Design review of the part built by this model. Coordinates are the model's own, in mm. A direction names the side the tool comes from. Coordinates: 2 decimals unless noted, no trailing zeros. Loops run counter-clockwise (first coordinate to the right, second up) from the corner with the lowest first, then second, coordinate; pieces in that order, holes last. Notation, with made-up numbers: M -8.5,-33.5 L 13.5,-33.5 A7 ccw 13.5,-25.5 Z; hole C 80,5.5 d6. An arc over 180 degrees is marked long. One line per item, written item: value.
```python
from build123d import *

# Parameters (mm, degrees)
F0_R     = 10.16
F1_DEPTH = 50.8
F3_R     = 3.175
F2_W     = 38.1
F2_H     = 15.875
F5_DEPTH = 31.751
F5_TAPER = 12
F6_DEPTH = 25.4


with BuildPart() as f1:
    # F0 (on Top) → F1 (new body)
    with BuildSketch(Plane.XY):
        with BuildLine():
            ThreePointArc((0, 15.875), (11.2253201513, 11.2253201513), (15.875, 0))
            ThreePointArc((15.875, 0), (15.8438414877, -0.9941387788), (15.7504882631, -1.9843750839))
            ThreePointArc((15.7504882631, -1.9843750839), (18.9005858967, 3.968749972), (25.2007812379, 6.35))
            Line((25.2007812379, 6.35), (47.625, 6.35))
            ThreePointArc((47.625, 6.35), (52.1151280605, 4.4901280605), (53.975, 0))
            Line((53.975, 0), (53.975, -12.7))
            ThreePointArc((53.975, -12.7), (54.9049359697, -14.9450640303), (57.15, -15.875))
            Line((57.15, -15.875), (60.325, -15.875))
            ThreePointArc((60.325, -15.875), (62.5700640303, -14.9450640303), (63.5, -12.7))
            Line((63.5, -12.7), (63.5, 3.175))
            ThreePointArc((63.5, 3.175), (59.7802561211, 12.1552561211), (50.8, 15.875))
            Line((50.8, 15.875), (0, 15.875))
        make_face()
        with BuildLine():
            ThreePointArc((15.7504882631, -1.9843750839), (15.8438414877, -0.9941387788), (15.875, 0))
            ThreePointArc((15.875, 0), (11.2253201513, 11.2253201513), (0, 15.875))
            ThreePointArc((0, 15.875), (-11.906250028, -10.5003254841), (15.7504882631, -1.9843750839))
        make_face()
        with Locations((0, 1.905)):
            Circle(F0_R, mode=Mode.SUBTRACT)
    extrude(amount=F1_DEPTH)

    # F3
    f3_edges = [f1.edges().sort_by_distance(p)[0] for p in [
        (25.4, 15.875, 0),
        (25.4, 15.875, 50.8),
    ]]
    fillet(f3_edges, radius=F3_R)

    # F2 (on face) → F5 (cut, through all)
    with BuildSketch(Plane(origin=(0, 15.875, 0), x_dir=(-1, 0, 0), z_dir=(0, 1, 0))):
        with BuildLine():
            ThreePointArc((-7.9375, 33.3375), (-15.875, 25.4), (-7.9375, 17.4625))
            Line((-7.9375, 17.4625), (0, 17.4625))
            Line((0, 17.4625), (0, 33.3375))
            Line((0, 33.3375), (-7.9375, 33.3375))
        make_face()
        with Locations((19.05, 25.4)):
            Rectangle(F2_W, F2_H)
    extrude(amount=-F5_DEPTH, taper=F5_TAPER, mode=Mode.SUBTRACT)

    # F4 (on face) → F6 (cut)
    with BuildSketch(Plane.XZ.offset(15.875)):
        with BuildLine():
            Line((-38.1, 21.828125), (7.9375, 21.828125))
            ThreePointArc((7.9375, 21.828125), (11.509375, 25.4), (7.9375, 28.971875))
            Line((7.9375, 28.971875), (-38.1, 28.971875))
            Line((-38.1, 28.971875), (-38.1, 21.828125))
        make_face()
    extrude(amount=-F6_DEPTH, mode=Mode.SUBTRACT)


solid = f1.part
```
(1) We need section A-A on x = 33. State the section outline as (y, z) points (3 decimals).
Reply:
outline: M 6.35,3.175 A3.175 ccw 9.525,0 L 12.7,0 A3.175 ccw 15.875,3.175 L 15.875,47.625 A3.175 ccw 12.7,50.8 L 9.525,50.8 A3.175 ccw 6.35,47.625 Z
(2) To check wall thickness, follow line 1 along Y through (x, z) = (0, 43) (3 decimals); line 2 along X through (y, z) = (-1, 48.5); line 3 along X through (y, z) = (-2, 6.5) (3 decimals). State the ranges of each line that lie inside material, in increasing order. Write a range as [from, to].
Reply:
line 1: y = [-15.875, -8.255], [12.065, 15.875]
line 2: x = [-15.72, -9.74], [9.74, 15.8], [54.1, 63.38]
line 3: x = [-15.749, -9.38], [9.38, 15.749], [53.975, 63.5]
(3) Tool access review of faces 1 (the cylindrical face through (4.688, -7.109, 10.761)), 2 (the cylindrical face through (54.88, -6.439, 49.845)), 3 (the flat face through (-3, -10, 28.972)), 4 (the cylindrical face through (36.57, 7.26, 0.95)), 5 (the flat face through (36, 6.35, 25)): name each direction out of +Z, -Z, +X, -X, +Y, -Y from which nothing blocks a thin tool from reaching the whole face with its end or side.
Reply:
face 1: +Z, -Z
face 2: +Z, -Y
face 3: -X, +Y, -Y
face 4: -Z, -Y
face 5: +Z, -Z, -Y
(4) We need section B-B on z = 40. State the section outline as (x, y) points (3 decimals).
Reply:
outline: M 0,15.875 A15.875 ccw long 15.75,-1.984 A9.525 cw 25.201,6.35 L 47.625,6.35 A6.35 cw 53.975,0 L 53.975,-12.7 A3.175 ccw 57.15,-15.875 L 60.325,-15.875 A3.175 ccw 63.5,-12.7 L 63.5,3.175 A12.7 ccw 50.8,15.875 Z; hole C 0,1.905 d20.32
(5) Insertion check: pin 1 (6.5 mm diameter, centred on y = -7, z = 18.5, fed in from -X); pin 2 (18.5 mm diameter, centred on x = 0, y = 1.905, fed in from -Z); pin 3 (9 mm diameter, centred on x = -7.5, y = -12, fed in from -Z); pin 4 (1 mm diameter, centred on y = -6.5, z = 23, fed in from -X). Each pin has a flat end and moves straight along its axis. Give the tip position at first contact, or say it passes through.
Reply:
pin 1: stops at x = -15.43
pin 2: passes through
pin 3: stops at z = 0
pin 4: stops at x = 10.02
(6) Mouldability with a two-part tool opening along X and no side actions: class faces 6 (the flat face through (26, 15.875, 25)), 7 (the cylindrical face through (18.829, 3.905, 25.089)), 8 (the cylindrical face through (62.59, -4.65, 49.85)) as released by +X, released by -X, zero draft, split by the parting line, or undercut.
Reply:
face 6: zero draft
face 7: undercut
face 8: released by +X
(7) We need section C-C on z = 25.4. State the section outline as (x, y) points (3 decimals).
Reply:
outline: M 11.509,-10.934 A15.875 ccw 15.75,-1.984 A9.525 cw 25.201,6.35 L 47.625,6.35 A6.35 cw 53.975,0 L 53.975,-12.7 A3.175 ccw 57.15,-15.875 L 60.325,-15.875 A3.175 ccw 63.5,-12.7 L 63.5,3.175 A12.7 ccw 50.8,15.875 L 15.875,15.875 L 11.509,-4.664 Z
(8) We need section D-D on x = -5. State how many separate pieces and enclosed holes the cut face has, then the cut area to 3 significant figures.
Reply:
separate pieces: 4
enclosed holes: 0
area: 502 mm2
